Verification items for the finished model (mm, model axes). A direction names the side the tool comes from. Give positions to 0.01 mm unless a question says otherwise; leave off trailing zeros. Write each loop counter-clockwise with the first axis right and the second up, starting at its lowest first coordinate (ties: lowest second). Pieces come first, ordered by that corner, then holes. Notation, with made-up numbers: (-37, 79.25) -> (-25, 79.25) arc R16 ccw to (-25, 100.25) -> close; hole circle Ø4 at (6, -0.75). An arc over 180 degrees is marked (long way). Answer as CSV lines item,"result".
```python
from build123d import *

# Parameters (mm, degrees)
BOSS_EXTRUDE1_DEPTH = 20
SKETCH2_R           = 2.4
SKETCH2_R_2         = 2.35
BOSS_EXTRUDE2_DEPTH = 3
CUT_EXTRUDE1_DEPTH  = 158.718007744
FILLET1_R           = 3.5


with BuildPart() as part:
    # Sketch1 → Boss-Extrude1 (new body)
    with BuildSketch(Plane(origin=(0, 0, 0), x_dir=(1, 0, 0), z_dir=(0, 1, 0))):
        Polygon((-57.597316241, 51.805869074), (-57.597316241, -8.444130926), (-46.097316241, -28.194130926), (-46.097316241, -108.194130926), (43.902683759, -108.194130926), (43.902683759, -28.194130926), (55.402683759, -8.444130926), (55.402683759, 51.805869074), align=None)
    extrude(amount=BOSS_EXTRUDE1_DEPTH)

    # Sketch2 → Boss-Extrude2 (add)
    with BuildSketch(Plane.XZ):
        with Locations(Location((-51.097316241, -45.305869074, 0), (0, 0, 90))):
            Circle(SKETCH2_R)
        with Locations(Location((48.902683759, -45.305869074, 0), (0, 0, 90))):
            Circle(SKETCH2_R)
        with Locations(Location((47.402683759, 6.944130926, 0), (0, 0, 90))):
            Circle(SKETCH2_R_2)
        with Locations(Location((-49.597316241, 6.944130926, 0), (0, 0, 90))):
            Circle(SKETCH2_R_2)
    extrude(amount=BOSS_EXTRUDE2_DEPTH)

    # Sketch3 → Cut-Extrude1 (cut, through all)
    with BuildSketch(Plane(origin=(55.402683759, 0, 0), x_dir=(0, 0, -1), z_dir=(1, 0, 0))):
        Polygon((-108.194130926, 20), (-108.194130926, 2.5), (-8.444130926, 13.563542172), (-8.444130926, 20), align=None)
        Polygon((-8.444130926, 20), (-8.444130926, 13.563542172), (49.587615005, 20), align=None)
        Polygon((49.587615005, 20), (51.805869074, 0), (51.805869074, 20), align=None)
    extrude(amount=-CUT_EXTRUDE1_DEPTH, mode=Mode.SUBTRACT)

    # Fillet1
    fillet1_edges = [part.edges().sort_by_distance(p)[0] for p in [
        (-57.597316241, 10, -50.69674204),
        (55.402683759, 10, -50.69674204),
        (-46.097316241, 5.686508139, 28.194130926),
        (-57.597316241, 6.781771086, 8.444130926),
        (43.902683759, 5.686508139, 28.194130926),
        (43.902683759, 1.25, 108.194130926),
        (-46.097316241, 1.25, 108.194130926),
        (55.402683759, 6.781771086, 8.444130926),
    ]]
    fillet(fillet1_edges, radius=FILLET1_R)


solid = part.part
```
1) Scan lines: line 1 along X through (y, z) = (3.75, 43.5); line 2 along Y through (x, z) = (-34.5, 27.5); line 3 along Y through (x, z) = (-37, 88). Record each from-to range of solid material in increasing order.
Reported:
line 1,"-46.1 to 43.9"
line 2,"0 to 11.45"
line 3,"0 to 4.74"
2) Section check A-A (x = -23). Record the boundary of the cut face in (y, z), and give its area (3 significant figures).
Reported:
outline,"(0, -51.81) -> (20, -49.59) -> (2.5, 108.19) -> (0, 108.19) -> close"
area,"1,800 mm²"
3) Draft check along Z on faces 1 (the flat face through (-0.36, 10.14, -50.68)), 2 (the flat face through (-46.097, 4, 58)), 3 (the cylindrical face through (-45.1, 1.46, 107.14)), 4 (the cylindrical face through (45.073, -1.479, 6.638)). Enter one of: +Z half, -Z half, draft (parallel to the pull), parting line (faces both ways), or undercut.
Reported:
face 1,"-Z half"
face 2,"draft"
face 3,"+Z half"
face 4,"undercut"
4) Section check B-B (z = 33). Record the boundary of the cut face in (x, y).
Reported:
outline,"(-46.1, 0) -> (43.9, 0) -> (43.9, 10.84) -> (-46.1, 10.84) -> close"
5) Tool access check on faces 5 (the cylindrical face through (-48.968, -1.479, -44.198)), 6 (the flat face through (43.903, 4, 59)), 7 (the flat face through (55.403, 7, -20)). Record the directions out of +Z, -Z, +X, -X, +Y, -Y that give a thin tool (end or side, any length) a straight path to the whole face; none if there is none.
Reported:
face 5,"-Y"
face 6,"+Z, +X, +Y, -Y"
face 7,"+Z, -Z, +X, +Y, -Y"
6) Section check C-C (z = -17). Record the boundary of the cut face in (x, y).
Reported:
outline,"(-57.6, 0) -> (55.4, 0) -> (55.4, 16.39) -> (-57.6, 16.39) -> close"
7) Depth check by flat-ended pin: pin 1 (5 mm diameter, centred on x = 2, z = -17, fed in from +Y); pin 2 (5.5 mm diameter, centred on y = 5, z = 61.5, fed in from -X); pin 3 (3 mm diameter, centred on x = -40, y = 17, fed in from -Z). Enter the tip coordinate at first touch or a pass-through.
Reported:
pin 1,"y = 16.66"
pin 2,"x = -46.1"
pin 3,"z = -50.09"
